Build history of the part. All positions in model axes, mm. A direction names the side the tool comes from. Coordinates: 2 decimals unless noted, no trailing zeros. Order: outer loops, then holes, each group sorted by start corner. A loop starts at its lowest first (then second) coordinate and runs counter-clockwise, first axis right, second up. Notation, with made-up numbers: (80, 44) - (109, 44) arc R15 cw to (109, 61) - close; hole circle Ø10 at (-28, 11). An arc over 180 degrees is marked (long way). One line per item, written item: value.
Autodesk Inventor part; units mm, degrees
ref_plane "YZ Plane" through (0, 0, 0) normal (1, 0, 0) x (0, 1, 0)
ref_plane "XZ Plane" through (0, 0, 0) normal (0, 1, 0) x (-1, 0, 0)
ref_plane "XY Plane" through (0, 0, 0) normal (0, 0, 1) x (1, 0, 0)
sketch "Sketch1" plane through (0, 0, 0) normal (0, 1, 0) x (-1, 0, 0)
  line L0 (0, 0) -> (-19.8882, 0)
  line L1 (-19.8882, 0) -> (-19.8882, -33.02)
  line L2 (-19.8882, -33.02) -> (0, -33.02)
  line L3 (0, -33.02) -> (0, 0)
  circle A0 centre (-12.9032, -3.048) radius 1.905
  circle A1 centre (-12.9032, -29.972) radius 1.905
  dimension "d0" = 19.8882
  dimension "d1" = 33.02
  dimension "d2" = 3.81
  dimension "d3" = 3.048
  dimension "d4" = 6.985
  dimension "d5" = 3.81
  dimension "d6" = 3.048
extrude "Extrusion1" add sketch "Sketch1" along normal blind 3.81
sketch "Sketch2" plane through (0, 3.81, 0) normal (0, 1, 0) x (1, 0, 0)
  circle A0 centre (5.1816, 13.208) radius 1.1938
  circle A1 centre (14.7066, 13.208) radius 1.1938
  circle A2 centre (12.9032, 3.048) radius 1.905
  point P0 (0, 0)
  dimension "d9" = 2.3876
  dimension "d10" = 2.3876
  dimension "d11" = 7.7216
  dimension "d12" = 1.8034
  dimension "d13" = 10.16
  dimension "d14" = 10.16
hole "Hole1" at (5.1816, 3.81, -13.208) at (14.7066, 3.81, -13.208) direction (0, -1, 0) diameter 2.3876 end through all counterbore diameter 5.08 counterbore depth 1.905
fillet "Fillet1" radius 3.175 4 edges at (19.8882, 1.905, -33.02) (0, 1.905, -33.02) (19.8882, 1.905, 0) (0, 1.905, 0)
properties part number "SwitchHolderTNutLeft"
1. Band-saw the part on B-B, the plane y = 0.8. Give the cut face in (x, z) (3 decimals).
Values found:
outline: (0, -29.845) arc R3.175 ccw to (3.175, -33.02) - (16.713, -33.02) arc R3.175 ccw to (19.888, -29.845) - (19.888, -3.175) arc R3.175 ccw to (16.713, 0) - (3.175, 0) arc R3.175 ccw to (0, -3.175) - close; hole circle Ø2.388 at (5.182, -13.208); hole circle Ø3.81 at (12.903, -29.972); hole circle Ø3.81 at (12.903, -3.048); hole circle Ø2.388 at (14.707, -13.208)
2. Probe line 1 along Z through (x, y) = (12.75, 1.05); line 2 along X through (y, z) = (2.9, -11.5); line 3 along Z through (x, y) = (13.25, 0.8). List the from-to ranges inside material, lowest first.
Values found:
line 1: z = -33.02 to -31.87, -28.07 to -4.95, -1.15 to 0
line 2: x = 0 to 3.3, 7.06 to 12.83, 16.59 to 19.89
line 3: z = -33.02 to -31.85, -28.1 to -4.92, -1.17 to 0
3. Band-saw the part on A-A, the plane z = -4. Give the cut face in (x, y), and give its area (3 significant figures).
Values found:
outline: (0, 0) - (11.25, 0) - (11.25, 3.81) - (0, 3.81) - close; (14.55, 0) - (19.89, 0) - (19.89, 3.81) - (14.55, 3.81) - close
area: 63.2 mm2
4. Band-saw the part on D-D, the plane y = 3.5. Give the cut face in (x, z) (3 decimals).
Values found:
outline: (0, -29.845) arc R3.175 ccw to (3.175, -33.02) - (16.713, -33.02) arc R3.175 ccw to (19.888, -29.845) - (19.888, -3.175) arc R3.175 ccw to (16.713, 0) - (3.175, 0) arc R3.175 ccw to (0, -3.175) - close; hole circle Ø5.08 at (5.182, -13.208); hole circle Ø3.81 at (12.903, -29.972); hole circle Ø3.81 at (12.903, -3.048); hole circle Ø5.08 at (14.707, -13.208)
5. Flat gauge pins, fed straight in: P1, Ø4, axis at x = 14.71, z = -13.21, coming from the +Y side (3 decimals); P2, Ø2, axis at x = 5.18, z = -13.21, coming from the -Y side. Where does each tip first touch, or does it go through?
Values found:
P1: stops at y = 1.905
P2: passes through
6. Two-plate mould, pull along Z, no slides. Class faces 1 (the face through (4.419, 2.844, -10.785)), 2 (the face through (18.98, 1.93, -32.07)), 3 (the face through (19.888, 2, -16)), 4 (the face through (16, 1.905, -14)): pulls with the +Z half, pulls with the -Z half, needs draft (parallel to the pull), parting line crosses it, or undercut.
Values found:
face 1: undercut
face 2: pulls with the -Z half
face 3: needs draft
face 4: undercut
7. Band-saw the part on C-C, the plane z = -11. Give the cut face in (x, y) (3 decimals).
Values found:
outline: (0, 0) - (19.888, 0) - (19.888, 3.81) - (15.962, 3.81) - (15.962, 1.905) - (13.451, 1.905) - (13.451, 3.81) - (6.437, 3.81) - (6.437, 1.905) - (3.926, 1.905) - (3.926, 3.81) - (0, 3.81) - close
8. 3-axis set-ups, long thin cutter, end or side, ignore diameter. For faces 5 (the face through (10, 2, -33.02)), 6 (the face through (6, 1.905, -12)): which of +Z, -Z, +X, -X, +Y, -Y reach the whole face in a straight line?
Values found:
face 5: -Z, +X, -X, +Y, -Y
face 6: +Y
